from build123d import *

# Parameters (mm, degrees)
SKETCH1_EXCAVATOR_MASTERSKETCH_3_R   = 2.25
SKETCH1_EXCAVATOR_MASTERSKETCH_3_R_2 = 14.2875
BOSS_EXTRUDE1_DEPTH                  = 1.5875


with BuildPart() as part:
    # Sketch1-Excavator Mastersketch_3 → Boss-Extrude1 (new body)
    with BuildSketch(Plane(origin=(101.6, 0, 0), x_dir=(0, 0, -1), z_dir=(1, 0, 0))):
        with BuildLine():
            Line((153.231778176, -25.4), (87.1, -25.4))
            ThreePointArc((87.1, -25.4), (85.332233047, -24.667766953), (84.6, -22.9))
            Line((84.6, -22.9), (84.6, 22.9))
            ThreePointArc((84.6, 22.9), (85.332233047, 24.667766953), (87.1, 25.4))
            Line((87.1, 25.4), (117.64344161, 25.4))
            ThreePointArc((117.64344161, 25.4), (118.600150191, 25.590301169), (119.411208563, 26.132233047))
            Line((119.411208563, 26.132233047), (143.357002179, 50.078026663))
            ThreePointArc((143.357002179, 50.078026663), (145.124769132, 50.81025971), (146.892536085, 50.078026663))
            Line((146.892536085, 50.078026663), (179.624035114, 17.346527635))
            ThreePointArc((179.624035114, 17.346527635), (180.341686112, 15.848385623), (179.961994288, 14.231200859))
            Line((179.961994288, 14.231200859), (155.337504304, -24.247559823))
            ThreePointArc((155.337504304, -24.247559823), (154.432007413, -25.093045777), (153.231778176, -25.4))
        make_face()
        with Locations((90.6, 19.4)):
            Circle(SKETCH1_EXCAVATOR_MASTERSKETCH_3_R, mode=Mode.SUBTRACT)
        with Locations((90.6, -19.4)):
            Circle(SKETCH1_EXCAVATOR_MASTERSKETCH_3_R, mode=Mode.SUBTRACT)
        with Locations((148.6, -19.4)):
            Circle(SKETCH1_EXCAVATOR_MASTERSKETCH_3_R, mode=Mode.SUBTRACT)
        with Locations((172.560512242, 15.924769132)):
            Circle(SKETCH1_EXCAVATOR_MASTERSKETCH_3_R, mode=Mode.SUBTRACT)
        with Locations((145.124769132, 43.360512242)):
            Circle(SKETCH1_EXCAVATOR_MASTERSKETCH_3_R, mode=Mode.SUBTRACT)
        with Locations((129.2, 0)):
            Circle(SKETCH1_EXCAVATOR_MASTERSKETCH_3_R_2, mode=Mode.SUBTRACT)
    extrude(amount=BOSS_EXTRUDE1_DEPTH)


solid = part.part
Work out the finished part from the listing and answer in its coordinate system (mm). Give positions to 0.01 mm unless a question says otherwise; leave off trailing zeros. Order: outer loops, then holes, each group sorted by start corner. A loop starts at its lowest first (then second) coordinate and runs counter-clockwise, first axis right, second up. Notation, with made-up numbers: (-3, 56) - (17, 56) arc R15 cw to (17, 64) - close; hole circle Ø9 at (-26, 32.5). An arc over 180 degrees is marked (long way). Answer as CSV lines item,"result". Start each with the question number.
Q1. Find the intervals of material crossed by L1, parallel to Y at x = 102.5, z = -90.6; L2, parallel to Y at x = 103.05, z = -94.5; L3, parallel to Z at x = 101.7, y = 17, in increasing order. Write a range as [from, to].
Q2. The mould has two halves that part along Y. Classify faces 1 (the face through (102.383, -18.724, -150.746)), 2 (the face through (102.383, 18.156, -172.268)), 3 (the face through (102.38, 33.94, -163.03)), 4 (the face through (102.383, -24.687, -85.352)): +Y half, -Y half, draft (parallel to the pull), parting line (faces both ways), or undercut.
Q3. The part is cut by section A-A (z = -90.6). Write down the section's boundary in (x, y).
Q4. Given pin 1 Ø4 at (y, z) = (-19.4, -148.6) entering from +X; pin 2 Ø7 at (y, z) = (-19.4, -90.6) entering from +X; pin 3 Ø0.5 at (x, z) = (102, -106) entering from +Y, each flat-ended and moving along its own axis, determine where each tip first touches the part or whether it passes through.
Q5. The part is cut by section D-D (z = -130). Write down the section's boundary in (x, y), then the cut area to 3 significant figures.
Q6. The part is cut by section C-C (y = -19.4). Write down the section's boundary in (x, z).
Q7. The part is cut by section B-B (y = -5). Write down the section's boundary in (x, z), then the cut area to 3 significant figures.
Check result:
1,L1,"y = [-25.4, -21.65], [-17.15, 17.15], [21.65, 25.4]"
1,L2,"y = [-25.4, 25.4]"
1,L3,"z = [-179.91, -174.54], [-170.58, -84.6]"
2,face 1,"undercut"
2,face 2,"undercut"
2,face 3,"+Y half"
2,face 4,"-Y half"
3,outline,"(101.6, -25.4) - (103.19, -25.4) - (103.19, -21.65) - (101.6, -21.65) - close; (101.6, -17.15) - (103.19, -17.15) - (103.19, 17.15) - (101.6, 17.15) - close; (101.6, 21.65) - (103.19, 21.65) - (103.19, 25.4) - (101.6, 25.4) - close"
4,pin 1,"passes through"
4,pin 2,"stops at x = 103.19"
4,pin 3,"stops at y = 25.4"
5,outline,"(101.6, -25.4) - (103.19, -25.4) - (103.19, -14.27) - (101.6, -14.27) - close; (101.6, 14.27) - (103.19, 14.27) - (103.19, 36.72) - (101.6, 36.72) - close"
5,area,"53.3 mm²"
6,outline,"(101.6, -158.44) - (103.19, -158.44) - (103.19, -150.85) - (101.6, -150.85) - close; (101.6, -146.35) - (103.19, -146.35) - (103.19, -92.85) - (101.6, -92.85) - close; (101.6, -88.35) - (103.19, -88.35) - (103.19, -84.6) - (101.6, -84.6) - close"
7,outline,"(101.6, -167.65) - (103.19, -167.65) - (103.19, -142.58) - (101.6, -142.58) - close; (101.6, -115.82) - (103.19, -115.82) - (103.19, -84.6) - (101.6, -84.6) - close"
7,area,"89.4 mm²"
